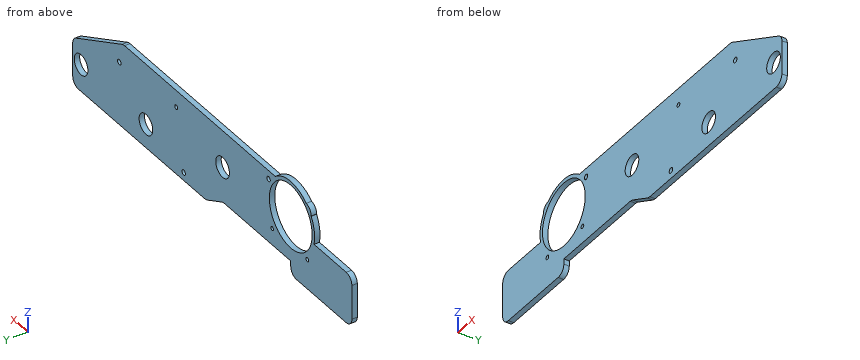
from build123d import *

# Parameters (mm, degrees)
SKETCH1_W           = 210
SKETCH1_H           = 50
SKETCH1_R           = 1.211665018
SKETCH1_R_2         = 1.165617118
SKETCH1_R_3         = 1.5
SKETCH1_R_4         = 1.25
SKETCH1_R_5         = 1.517273905
BOSS_EXTRUDE1_DEPTH = 3.175
SKETCH2_R           = 2
CUT_EXTRUDE1_DEPTH  = 10
SKETCH3_R           = 6
SKETCH3_R_2         = 0.586995366
CUT_EXTRUDE2_DEPTH  = 57.15
CUT_EXTRUDE7_DEPTH  = 10
FILLET3_R           = 5
SKETCH11_R          = 18.5
SKETCH11_R_2        = 2
BOSS_EXTRUDE4_DEPTH = 3.175
SKETCH12_R          = 21
BOSS_EXTRUDE5_DEPTH = 3.175
SKETCH13_R          = 18.85
CUT_EXTRUDE8_DEPTH  = 3.175
BOSS_EXTRUDE6_DEPTH = 3.175
FILLET4_R           = 5


with BuildPart() as part:
    # Sketch1 → Boss-Extrude1 (new body)
    with BuildSketch(Plane(origin=(0, 0, 0), x_dir=(1, 0, 0), z_dir=(0, 1, 0))):
        with Locations((105, -25)):
            Rectangle(SKETCH1_W, SKETCH1_H)
        with Locations(Location((3.489526233, -16.787661112, 0), (0, 0, 270))):
            Circle(SKETCH1_R, mode=Mode.SUBTRACT)
        with Locations(Location((34.37258772, -17.194005245, 0), (0, 0, 270))):
            Circle(SKETCH1_R_2, mode=Mode.SUBTRACT)
        with Locations(Location((37.520749958, -44.921198121, 0), (0, 0, 270))):
            Circle(SKETCH1_R_3, mode=Mode.SUBTRACT)
        with Locations(Location((118.879039361, -40.017685043, 0), (0, 0, 270))):
            Circle(SKETCH1_R_4, mode=Mode.SUBTRACT)
        with Locations(Location((112.302052499, -4.739260115, 0), (0, 0, 270))):
            Circle(SKETCH1_R_3, mode=Mode.SUBTRACT)
        with Locations(Location((168.975233936, -37.403209633, 0), (0, 0, 270))):
            Circle(SKETCH1_R_5, mode=Mode.SUBTRACT)
    extrude(amount=BOSS_EXTRUDE1_DEPTH)

    # Sketch2 → Cut-Extrude1 (cut)
    with BuildSketch(Plane(origin=(0, 3.175, 0), x_dir=(1, 0, 0), z_dir=(0, 1, 0))):
        with Locations(Location((10, -26, 0), (0, 0, 270))):
            Circle(SKETCH2_R)
        with Locations(Location((10, -42, 0), (0, 0, 270))):
            Circle(SKETCH2_R)
        with Locations(Location((26, -26, 0), (0, 0, 270))):
            Circle(SKETCH2_R)
        with Locations(Location((26, -42, 0), (0, 0, 270))):
            Circle(SKETCH2_R)
    extrude(amount=-CUT_EXTRUDE1_DEPTH, mode=Mode.SUBTRACT)

    # Sketch3 → Cut-Extrude2 (cut)
    with BuildSketch(Plane(origin=(0, 3.175, 0), x_dir=(1, 0, 0), z_dir=(0, 1, 0))):
        with Locations(Location((78.01026379, -28.1, 0), (0, 0, 270))):
            Circle(SKETCH3_R)
        with Locations(Location((145.531297368, -14, 0), (0, 0, 270))):
            Circle(SKETCH3_R)
        with Locations(Location((18, -34, 0), (0, 0, 270))):
            Circle(SKETCH3_R_2)
        with Locations(Location((202.646291021, -16, 0), (0, 0, 270))):
            Circle(SKETCH3_R)
    extrude(amount=-CUT_EXTRUDE2_DEPTH, mode=Mode.SUBTRACT)

    # Sketch10 → Cut-Extrude7 (cut)
    with BuildSketch(Plane(origin=(0, 3.175, 0), x_dir=(1, 0, 0), z_dir=(0, 1, 0))):
        Polygon((210, -27.859435908), (165.502877994, -50), (210, -50), align=None)
        Polygon((92.532613397, 0), (77.65477062, -7.402812063), (0, -7.402812063), (0, 0), align=None)
    extrude(amount=-CUT_EXTRUDE7_DEPTH, mode=Mode.SUBTRACT)

    # Fillet3
    fillet3_edges = [part.edges().sort_by_distance(p)[0] for p in [
        (210, 1.5875, 0),
        (0, 1.5875, 50),
        (92.532613397, 1.5875, 0),
        (210, 1.5875, 27.859435908),
        (165.502877994, 1.5875, 50),
        (77.65477062, 1.5875, 7.402812063),
        (0, 1.5875, 7.402812063),
    ]]
    fillet(fillet3_edges, radius=FILLET3_R)

    # Sketch11 → Boss-Extrude4 (add)
    with BuildSketch(Plane(origin=(0, 3.175, 0), x_dir=(1, 0, 0), z_dir=(0, 1, 0))):
        with Locations((18, -34)):
            Circle(SKETCH11_R)
        with Locations(Location((10, -26, 0), (0, 0, 270))):
            Circle(SKETCH11_R_2, mode=Mode.SUBTRACT)
        with Locations(Location((10, -42, 0), (0, 0, 270))):
            Circle(SKETCH11_R_2, mode=Mode.SUBTRACT)
        with Locations(Location((26, -26, 0), (0, 0, 270))):
            Circle(SKETCH11_R_2, mode=Mode.SUBTRACT)
        with Locations(Location((26, -42, 0), (0, 0, 270))):
            Circle(SKETCH11_R_2, mode=Mode.SUBTRACT)
    extrude(amount=-BOSS_EXTRUDE4_DEPTH)

    # Sketch12 → Boss-Extrude5 (add)
    with BuildSketch(Plane(origin=(0, 3.175, 0), x_dir=(1, 0, 0), z_dir=(0, 1, 0))):
        with Locations((18, -34)):
            Circle(SKETCH12_R)
    extrude(amount=-BOSS_EXTRUDE5_DEPTH)

    # Sketch13 → Cut-Extrude8 (cut)
    with BuildSketch(Plane(origin=(0, 3.175, 0), x_dir=(1, 0, 0), z_dir=(0, 1, 0))):
        with Locations(Location((18, -34, 0), (0, 0, 270))):
            Circle(SKETCH13_R)
    extrude(amount=-CUT_EXTRUDE8_DEPTH, mode=Mode.SUBTRACT)

    # Sketch14 → Boss-Extrude6 (add)
    with BuildSketch(Plane(origin=(0, 3.175, 0), x_dir=(1, 0, 0), z_dir=(0, 1, 0))):
        with BuildLine():
            Line((-35.83, -29.449062132), (-2.500950332, -29.449062132))
            ThreePointArc((-2.500950332, -29.449062132), (-1.503732803, -26.215116779), (0, -23.183346174))
            Line((0, -23.183346174), (0, -12.402812063))
            Line((0, -12.402812063), (0, -12.248529085))
            Line((0, -12.248529085), (0, 0.727187937))
            Line((0, 0.727187937), (-35.83, 0.727187937))
            Line((-35.83, 0.727187937), (-35.83, -29.449062132))
        make_face()
        with BuildLine():
            Line((0, 0.727187937), (0, -12.248529085))
            Line((0, -12.248529085), (0.002380891, -12.248529085))
            ThreePointArc((0.002380891, -12.248529085), (1.51944077, -8.813145304), (5, -7.402812063))
            Line((5, -7.402812063), (18, -7.402812063))
            Line((18, -7.402812063), (18, 0.727187937))
            Line((18, 0.727187937), (0, 0.727187937))
        make_face()
    extrude(amount=-BOSS_EXTRUDE6_DEPTH)

    # Fillet4
    fillet4_edges = [part.edges().sort_by_distance(p)[0] for p in [
        (-35.83, 1.5875, 29.449062132),
        (-35.83, 1.5875, -0.727187937),
        (18, 1.5875, -0.727187937),
    ]]
    fillet(fillet4_edges, radius=FILLET4_R)


solid = part.part
Model file for the job. Use its own axes, mm. Coordinates: 2 decimals unless noted, no trailing zeros. Write each loop counter-clockwise with the first axis right and the second up, starting at its lowest first coordinate (ties: lowest second). Pieces come first, ordered by that corner, then holes. Notation, with made-up numbers: (16.25, 84) -> (65.25, 84) arc R33 cw to (65.25, 122) -> close; hole circle Ø3 at (68, 61.25). An arc over 180 degrees is marked (long way). One line per item, written item: value. Start each with the question number.
1) Slice it at B-B on x = -19. Write the cut outline in (y, z) (3 decimals).
2) Flat gauge pins, fed straight in: pin 1 Ø1.9 at (x, z) = (3.49, 16.79) entering from +Y; pin 2 Ø1 at (x, y) = (41, 2.5) entering from -Z; pin 3 Ø1.5 at (y, z) = (1, 34.5) entering from -X; pin 4 Ø15.5 at (x, z) = (145.53, 14) entering from -Y. Where does each tip first touch, or does it go through?
3) Slice it at C-C on x = 180.5. Write the cut outline in (y, z) (3 decimals).
4) Probe probe 1 along X at (y, z) = (1.8, 21.5); probe 2 along X at (y, z) = (3.05, 44); probe 3 along Z at (x, y) = (4.5, 1.85). List the from-to ranges inside material, lowest first.
Answers follow:
1. outline: (0, -0.727) -> (3.175, -0.727) -> (3.175, 29.449) -> (0, 29.449) -> close
2. pin 1: through
2. pin 2: z = 7.4
2. pin 3: x = -3
2. pin 4: y = 0
3. outline: (0, 0) -> (3.175, 0) -> (3.175, 42.538) -> (0, 42.538) -> close
4. probe 1: -35.83 to 3.89, 32.11 to 200.25, 205.04 to 210
4. probe 2: -0.47 to 2.02, 33.98 to 36.47, 38.7 to 177.56
4. probe 3: -0.73 to 16.12, 17.46 to 20.84, 47.16 to 50.09
